The model under review builds one solid part; all positions refer to its coordinate system, in mm. Face numbers are marked on the shaded views. A direction names the side the tool comes from. Give positions to 0.01 mm unless a question says otherwise; leave off trailing zeros. Order: outer loops, then holes, each group sorted by start corner. A loop starts at its lowest first (then second) coordinate and runs counter-clockwise, first axis right, second up.
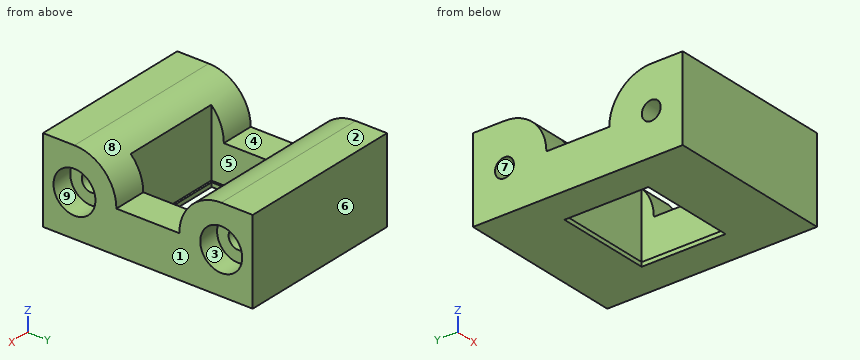
```python
from build123d import *

# Parameters (mm, degrees)
SKETCH_W        = 40
SKETCH_H        = 50
SKETCH_W_2      = 23
SKETCH_H_2      = 20
PAD_DEPTH       = 20
SKETCH001_R     = 2.25
POCKET_DEPTH    = 40.001
SKETCH002_W     = 24
SKETCH002_H     = 21
POCKET001_DEPTH = 19
SKETCH003_R     = 5
POCKET002_DEPTH = 5
POCKET003_DEPTH = 40.001


with BuildPart() as part:
    # Sketch → Pad (new body)
    with BuildSketch(Plane.XY):
        with Locations((20, 25)):
            Rectangle(SKETCH_W, SKETCH_H)
        with Locations((20, 25)):
            Rectangle(SKETCH_W_2, SKETCH_H_2, mode=Mode.SUBTRACT)
    extrude(amount=PAD_DEPTH)

    # Sketch001 → Pocket (cut, through all)
    with BuildSketch(Plane.YZ.offset(40)):
        with Locations((7.5, 10)):
            Circle(SKETCH001_R)
        with Locations((42.5, 10)):
            Circle(SKETCH001_R)
    extrude(amount=-POCKET_DEPTH, mode=Mode.SUBTRACT)

    # Sketch002 → Pocket001 (cut)
    with BuildSketch(Plane.XY.offset(20)):
        with Locations((20, 25)):
            Rectangle(SKETCH002_W, SKETCH002_H)
    extrude(amount=-POCKET001_DEPTH, mode=Mode.SUBTRACT)

    # Sketch003 → Pocket002 (cut)
    with BuildSketch(Plane.YZ.offset(40)):
        with Locations((7.5, 10)):
            Circle(SKETCH003_R)
        with Locations((42.5, 10)):
            Circle(SKETCH003_R)
    extrude(amount=-POCKET002_DEPTH, mode=Mode.SUBTRACT)

    # Sketch004 → Pocket003 (cut, through all)
    with BuildSketch(Plane.YZ.offset(40)):
        with BuildLine():
            ThreePointArc((17.5, 10), (14.571068, 17.071068), (7.5, 20))
            Line((7.5, 20), (7.5, 22))
            Line((7.5, 22), (42.5, 22))
            Line((42.5, 22), (42.5, 20))
            ThreePointArc((42.5, 20), (35.428932, 17.071068), (32.5, 10))
            Line((32.5, 10), (17.5, 10))
        make_face()
    extrude(amount=-POCKET003_DEPTH, mode=Mode.SUBTRACT)


solid = part.part
```
Item 1: Take a section at A-A (x = 28). Give the boundary of the cut face in (y, z), and give its area (3 significant figures).
Values found:
outline: (0, 0) - (15, 0) - (15, 1) - (14.5, 1) - (14.5, 17.14) arc R10 ccw to (7.5, 20) - (0, 20) - close; (35, 0) - (50, 0) - (50, 20) - (42.5, 20) arc R10 ccw to (35.5, 17.14) - (35.5, 1) - (35, 1) - close; hole circle Ø4.5 at (7.5, 10); hole circle Ø4.5 at (42.5, 10)
area: 537 mm2
Item 2: Take a section at D-D (x = 5). Give the boundary of the cut face in (y, z).
Values found:
outline: (0, 0) - (50, 0) - (50, 20) - (42.5, 20) arc R10 ccw to (32.5, 10) - (17.5, 10) arc R10 ccw to (7.5, 20) - (0, 20) - close; hole circle Ø4.5 at (7.5, 10); hole circle Ø4.5 at (42.5, 10)
Item 3: Take a section at B-B (z = 4.25). Give the boundary of the cut face in (x, y).
Values found:
outline: (0, 0) - (40, 0) - (40, 50) - (0, 50) - close; hole (8, 14.5) - (32, 14.5) - (32, 35.5) - (8, 35.5) - close
Item 4: Take a section at C-C (y = 16.5). Give the boundary of the cut face in (x, z), and give its area (3 significant figures).
Values found:
outline: (0, 0) - (8.5, 0) - (8.5, 1) - (8, 1) - (8, 14.36) - (0, 14.36) - close; (31.5, 0) - (40, 0) - (40, 14.36) - (32, 14.36) - (32, 1) - (31.5, 1) - close
area: 231 mm2
Item 5: For line 1 (Z direction, x = 37.25, y = 42.5); line 2 (Y direction, x = 21.5, z = 4.25); line 3 (X direction, y = 31, z = 7), list the stretches that pass through material, from the lowest coordinate up.
Values found:
line 1: z = 0 to 5, 15 to 20
line 2: y = 0 to 14.5, 35.5 to 50
line 3: x = 0 to 8, 32 to 40
Item 6: Draft analysis for pull direction Z (two halves, no side actions). For the marked faces 6, 7, 8 and 9, state which applies: released by +Z, released by -Z, zero draft, split by the parting line, or undercut.
Values found:
face 6: zero draft
face 7: undercut
face 8: released by +Z
face 9: undercut
Item 7: For the marked faces 1, 2, 3, 4 and 5, list the 3-axis set-ups (+Z, -Z, +X, -X, +Y, -Y) from which the entire face can be reached by the end or side of a thin tool; tool diameter is ignored.
Values found:
face 1: +Z, -Z, +X, +Y, -Y
face 2: +Z, +X, -X, +Y, -Y
face 3: +X
face 4: +Z, +X, -X
face 5: +Z
Item 8: Clearance check with flat-ended pins moving along their axes: pin 1 Ø3 at (x, y) = (35, 32) entering from +Z; pin 2 Ø2.5 at (y, z) = (7.5, 10) entering from -X; pin 3 Ø6.5 at (x, y) = (3.5, 24) entering from +Z; pin 4 Ø3 at (y, z) = (5.5, 12) entering from +X. State where each tip first meets the part, or that it passes through.
Values found:
pin 1: stops at z = 14.36
pin 2: passes through
pin 3: stops at z = 10
pin 4: stops at x = 35
